Check sheet for the modelled part. Datum: model origin and axes. Units: mm. A direction names the side the tool comes from. Round coordinates to 2 decimals unless told otherwise and drop trailing zeros. Write each loop counter-clockwise with the first axis right and the second up, starting at its lowest first coordinate (ties: lowest second). Pieces come first, ordered by that corner, then holes.
Item 1: Go/stop test with flat-tipped pins: pin 1 Ø16 at (x, z) = (-50, 24.5) entering from +Y; pin 2 Ø5 at (x, y) = (-55, -21.5) entering from -Z; pin 3 Ø6 at (x, y) = (-34, 20.5) entering from -Z. Record where each tip stops, or that it passes through.
Item 2: Cross-section at A-A on z = -7.5. Enter the section's corners in (x, y), plus the area to 3 significant figures.
Item 3: Material ranges on line 1 (X direction, y = -18, z = -1); line 2 (Z direction, x = -7.5, y = 21); line 3 (Y direction, x = -56, z = 19.5), recorded low to high.
Item 4: Tool access check on faces 1 (the cylindrical face through (17.27, 7.75, -5.92)), 2 (the flat face through (34, -22, 20)), 3 (the flat face through (34, -22, -5)), 4 (the flat face through (-51, -16.75, -5)), 5 (the flat face through (51, -16.75, 20)). Record the directions out of +Z, -Z, +X, -X, +Y, -Y that give a thin tool (end or side, any length) a straight path to the whole face; none if there is none.
Item 5: Cross-section at D-D on x = 40. Enter the section's corners in (y, z).
Item 6: Cross-section at B-B on x = 12.5. Enter the section's corners in (y, z).
Item 7: Cross-section at C-C on y = 9.25. Enter the section's corners in (x, z), plus the area to 3 significant figures.
Item 8: Release check for a two-part mould opening along X. For faces 6 (the flat face through (1, -26.75, 9.7)), 7 (the flat face through (-68, -6, 5)), 8 (the flat face through (68, -6, 5)), 9 (the flat face through (-34, -22, -5)) record: +X half, -X half, draft (parallel to the pull), parting line (faces both ways), or undercut.
from build123d import *

# Parameters (mm, degrees)
SKETCH1_W           = 136
SKETCH1_H           = 53.5
BOSS_EXTRUDE1_DEPTH = 10
SKETCH2_R           = 5
BOSS_EXTRUDE2_DEPTH = 12
SKETCH3_W           = 10
SKETCH3_H           = 10
SKETCH3_W_2         = 20
BOSS_EXTRUDE3_DEPTH = 34


with BuildPart() as part:
    # Sketch1 → Boss-Extrude1 (new body)
    with BuildSketch(Plane.XY):
        Rectangle(SKETCH1_W, SKETCH1_H)
    extrude(amount=BOSS_EXTRUDE1_DEPTH)

    # Sketch2 → Boss-Extrude2 (add)
    with BuildSketch(Plane(origin=(0, 0, 0), x_dir=(-1, 0, 0), z_dir=(0, 0, -1))):
        with Locations(Location((12.5, 9.25, 0), (0, 0, 180))):
            Circle(SKETCH2_R)
        with Locations(Location((-12.5, 9.25, 0), (0, 0, 180))):
            Circle(SKETCH2_R)
    extrude(amount=BOSS_EXTRUDE2_DEPTH)

    # Sketch3 → Boss-Extrude3 (add)
    with BuildSketch(Plane.ZY.offset(68)):
        with Locations((-5, -21.75)):
            Rectangle(SKETCH3_W, SKETCH3_H)
        with Locations((20, -21.75)):
            Rectangle(SKETCH3_W_2, SKETCH3_H)
    boss_extrude3 = extrude(amount=-BOSS_EXTRUDE3_DEPTH)

    # Mirror2: Boss-Extrude3 across plane
    add(boss_extrude3.mirror(Plane.ZY))


solid = part.part
Response values:
1. pin 1: stops at y = -16.75
1. pin 2: stops at z = -10
1. pin 3: stops at z = 0
2. outline: (-68, -26.75) - (-34, -26.75) - (-34, -16.75) - (-68, -16.75) - close; circle Ø10 at (-12.5, 9.25); circle Ø10 at (12.5, 9.25); (34, -26.75) - (68, -26.75) - (68, -16.75) - (34, -16.75) - close
2. area: 837 mm2
3. line 1: x = -68 to -34, 34 to 68
3. line 2: z = 0 to 10
3. line 3: y = -26.75 to -16.75
4. face 1: -Z
4. face 2: +Z, +Y, -Y
4. face 3: -Z, +Y, -Y
4. face 4: -Z, +X, -X, +Y
4. face 5: +Z, +X, -X, +Y
5. outline: (-26.75, -10) - (-16.75, -10) - (-16.75, 0) - (26.75, 0) - (26.75, 10) - (-16.75, 10) - (-16.75, 30) - (-26.75, 30) - close
6. outline: (-26.75, 0) - (4.25, 0) - (4.25, -12) - (14.25, -12) - (14.25, 0) - (26.75, 0) - (26.75, 10) - (-26.75, 10) - close
7. outline: (-68, 0) - (-17.5, 0) - (-17.5, -12) - (-7.5, -12) - (-7.5, 0) - (7.5, 0) - (7.5, -12) - (17.5, -12) - (17.5, 0) - (68, 0) - (68, 10) - (-68, 10) - close
7. area: 1,600 mm2
8. face 6: draft
8. face 7: -X half
8. face 8: +X half
8. face 9: undercut
